The listing builds one solid part. Answer for the finished solid, in the listing's coordinates (mm). Face numbers are marked on the shaded views. A direction names the side the tool comes from. Round coordinates to 2 decimals unless told otherwise and drop trailing zeros. Write each loop counter-clockwise with the first axis right and the second up, starting at its lowest first coordinate (ties: lowest second). Pieces come first, ordered by that corner, then holes. Notation, with made-up numbers: (50.5, 1.5) - (57.5, 1.5) arc R37 ccw to (57.5, 40.5) - close; hole circle Ø11 at (19.25, 75). An arc over 180 degrees is marked (long way). Answer in a Markdown table with one row per item.
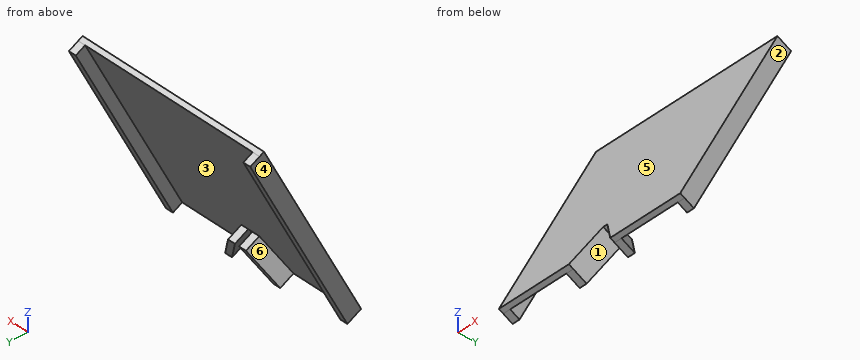
from build123d import *

# Parameters (mm, degrees)
BOSS_EXTRUDE1_DEPTH = 1317.1
CUT_EXTRUDE3_DEPTH  = 1956.361044318
SKETCH8_W           = 50
SKETCH8_H           = 1431.6
BOSS_EXTRUDE3_DEPTH = 70
BOSS_EXTRUDE4_DEPTH = 100


with BuildPart() as part:
    # Sketch1 → Boss-Extrude1 (new body)
    with BuildSketch(Plane(origin=(0, 0, 0), x_dir=(0, 0, -1), z_dir=(1, 0, 0))):
        Polygon((0, 0), (1275.564940028, -649.932799427), (1290.592025569, -620.440483477), (15.027085541, 29.492315951), align=None)
    extrude(amount=BOSS_EXTRUDE1_DEPTH)

    # Sketch6 → Cut-Extrude3 (cut, through all)
    with BuildSketch(Plane(origin=(0, 29.492315951, -15.027085541), x_dir=(1, 0, 0), z_dir=(0, 0.8910065241883676, -0.45399049973954747))):
        Polygon((808.5, 1431.6), (508.5, 1431.6), (643.5, 1200), (673.5, 1200), align=None)
    extrude(amount=-CUT_EXTRUDE3_DEPTH, mode=Mode.SUBTRACT)

    # Sketch8 → Boss-Extrude3 (add)
    with BuildSketch(Plane(origin=(0, 29.492315951, -15.027085541), x_dir=(1, 0, 0), z_dir=(0, 0.8910065241883676, -0.45399049973954747))):
        with Locations((25, 715.8)):
            Rectangle(SKETCH8_W, SKETCH8_H)
        with Locations((1292.1, 715.8)):
            Rectangle(SKETCH8_W, SKETCH8_H)
    extrude(amount=BOSS_EXTRUDE3_DEPTH)

    # Sketch8<4> → Boss-Extrude4 (add)
    with BuildSketch(Plane(origin=(0, 29.492315951, -15.027085541), x_dir=(1, 0, 0), z_dir=(0, 0.8910065241883676, -0.45399049973954747))):
        Polygon((808.5, 1431.6), (673.5, 1200), (723.5, 1200), (858.5, 1431.6), align=None)
        Polygon((458.6, 1431.6), (593.6, 1200), (643.5, 1200), (508.5, 1431.6), align=None)
    extrude(amount=BOSS_EXTRUDE4_DEPTH)


solid = part.part
(1) Section B-B (y = -326.5) is taken. Give the vertices of the cut face in (x, z), and give its area (3 significant figures).
Checked values:
| item | result |
|---|---|
| outline | (0, -867.89) - (50, -867.89) - (50, -713.7) - (1267.1, -713.7) - (1267.1, -867.89) - (1317.1, -867.89) - (1317.1, -640.79) - (0, -640.79) - close |
| area | 111,000 mm2 |
(2) Flat-ended cylindrical pins translate along their axes: pin 1 (6 mm diameter, centred on x = 256, y = -87.5, fed in from +Z); pin 2 (4 mm diameter, centred on x = 472, z = -837.5, fed in from +Y); pin 3 (8 mm diameter, centred on x = 167, z = -208, fed in from +Y). Find the tip coordinate at first contact, or state that the pin passes through.
Checked values:
| item | result |
|---|---|
| pin 1 | stops at z = -165.84 |
| pin 2 | stops at y = -388.56 |
| pin 3 | stops at y = -66.79 |
(3) For the marked faces 1 and 2, determine the directions among +Z, -Z, +X, -X, +Y, -Y from which every point of the face is accessible in a straight line to the end or side of a thin tool.
Checked values:
| item | result |
|---|---|
| face 1 | -Z, -Y |
| face 2 | +Z, -Z, +X, +Y, -Y |
(4) Find the intervals of material crossed by line 1 (X direction, y = -428, z = -960.5); line 2 (Z direction, x = 1109.5, y = -468); line 3 (Y direction, x = 763.5, z = -732.5), in increasing order.
Checked values:
| item | result |
|---|---|
| line 1 | x = 0 to 50, 1267.1 to 1317.1 |
| line 2 | z = -991.41 to -918.5 |
| line 3 | y = -373.23 to -336.08 |
(5) Section A-A (z = -1198.5) is taken. Give the vertices of the cut face in (x, y), and give its area (3 significant figures).
Checked values:
| item | result |
|---|---|
| outline | (0, -610.67) - (558.92, -610.67) - (598.45, -461.28) - (548.55, -461.28) - (518.85, -573.52) - (50, -573.52) - (50, -494.95) - (0, -494.95) - close; (718.55, -461.28) - (758.08, -610.67) - (1317.1, -610.67) - (1317.1, -494.95) - (1267.1, -494.95) - (1267.1, -573.52) - (798.25, -573.52) - (768.55, -461.28) - close |
| area | 61,000 mm2 |
(6) Section C-C (z = -487) is taken. Give the vertices of the cut face in (x, y).
Checked values:
| item | result |
|---|---|
| outline | (0, -248.14) - (1317.1, -248.14) - (1317.1, -132.43) - (1267.1, -132.43) - (1267.1, -210.99) - (50, -210.99) - (50, -132.43) - (0, -132.43) - close |
(7) Section D-D (x = 939) is taken. Give the vertices of the cut face in (y, z), and give its area (3 significant figures).
Checked values:
| item | result |
|---|---|
| outline | (-649.93, -1275.56) - (-620.44, -1290.59) - (29.49, -15.03) - (0, 0) - close |
| area | 47,400 mm2 |
(8) For a pull along X with two mould halves and no side action, classify the marked faces 3, 4, 5 and 6 as pulls with the +X half, pulls with the -X half, needs draft (parallel to the pull), parting line crosses it, or undercut.
Checked values:
| item | result |
|---|---|
| face 3 | undercut |
| face 4 | pulls with the -X half |
| face 5 | needs draft |
| face 6 | undercut |
